```python
from build123d import *

# Parameters (mm, degrees)
SKETCH1_R           = 150
BOSS_EXTRUDE1_DEPTH = 9.52
SKETCH2_R           = 15.5
CUT_EXTRUDE1_DEPTH  = 213.345544808
SKETCH3_R           = 17.505
CUT_EXTRUDE2_DEPTH  = 8
SKETCH4_R           = 2.5
SKETCH4_R_2         = 1.65
CUT_EXTRUDE3_DEPTH  = 213.345544808
SKETCH6_R           = 1.65
CUT_EXTRUDE5_DEPTH  = 213.345544808
SKETCH7_R           = 4.5
CUT_EXTRUDE6_DEPTH  = 213.345544808


with BuildPart() as part:
    # Sketch1 → Boss-Extrude1 (new body)
    with BuildSketch(Plane(origin=(0, 0, 0), x_dir=(1, 0, 0), z_dir=(0, 1, 0))):
        with Locations(Location((0, 0, 0), (0, 0, 270))):
            Circle(SKETCH1_R)
    extrude(amount=BOSS_EXTRUDE1_DEPTH)

    # Sketch2 → Cut-Extrude1 (cut, through all)
    with BuildSketch(Plane(origin=(0, 9.52, 0), x_dir=(1, 0, 0), z_dir=(0, 1, 0))):
        with Locations(Location((0, 0, 0), (0, 0, 270))):
            Circle(SKETCH2_R)
    extrude(amount=-CUT_EXTRUDE1_DEPTH, mode=Mode.SUBTRACT)

    # Sketch3 → Cut-Extrude2 (cut)
    with BuildSketch(Plane(origin=(0, 9.52, 0), x_dir=(1, 0, 0), z_dir=(0, 1, 0))):
        with Locations(Location((0, 0, 0), (0, 0, 270))):
            Circle(SKETCH3_R)
    extrude(amount=-CUT_EXTRUDE2_DEPTH, mode=Mode.SUBTRACT)

    # Sketch4 → Cut-Extrude3 (cut, through all)
    with BuildSketch(Plane(origin=(0, 9.52, 0), x_dir=(1, 0, 0), z_dir=(0, 1, 0))):
        with Locations(Location((10.725147849, -21.193217308, 0), (0, 0, 270))):
            Circle(SKETCH4_R)
        with Locations(Location((-23.716438501, 1.308358157, 0), (0, 0, 270))):
            Circle(SKETCH4_R)
        with Locations(Location((12.991290652, 19.884859151, 0), (0, 0, 270))):
            Circle(SKETCH4_R)
        with Locations(Location((67.75, -117.346442213, 0), (0, 0, 270))):
            Circle(SKETCH4_R_2)
        with Locations(Location((0, -135.5, 0), (0, 0, 270))):
            Circle(SKETCH4_R_2)
        with Locations(Location((-67.75, -117.346442213, 0), (0, 0, 270))):
            Circle(SKETCH4_R_2)
        with Locations(Location((-117.346442213, -67.75, 0), (0, 0, 270))):
            Circle(SKETCH4_R_2)
        with Locations(Location((-135.5, 0, 0), (0, 0, 270))):
            Circle(SKETCH4_R_2)
        with Locations(Location((-117.346442213, 67.75, 0), (0, 0, 270))):
            Circle(SKETCH4_R_2)
        with Locations(Location((-67.75, 117.346442213, 0), (0, 0, 270))):
            Circle(SKETCH4_R_2)
        with Locations(Location((0, 135.5, 0), (0, 0, 270))):
            Circle(SKETCH4_R_2)
        with Locations(Location((67.75, 117.346442213, 0), (0, 0, 270))):
            Circle(SKETCH4_R_2)
        with Locations(Location((117.346442213, 67.75, 0), (0, 0, 270))):
            Circle(SKETCH4_R_2)
        with Locations(Location((135.5, 0, 0), (0, 0, 270))):
            Circle(SKETCH4_R_2)
        with Locations(Location((117.346442213, -67.75, 0), (0, 0, 270))):
            Circle(SKETCH4_R_2)
    extrude(amount=-CUT_EXTRUDE3_DEPTH, mode=Mode.SUBTRACT)

    # Sketch6 → Cut-Extrude5 (cut, through all)
    with BuildSketch(Plane(origin=(0, 0, 0), x_dir=(-1, 0, 0), z_dir=(0, -1, 0))):
        with Locations(Location((-63.964762127, 126.790217897, 0), (0, 0, 90))):
            Circle(SKETCH6_R)
        with Locations(Location((-77.821168587, 118.790217897, 0), (0, 0, 90))):
            Circle(SKETCH6_R)
        with Locations(Location((-64.892965357, 112.397913052, 0), (0, 0, 90))):
            Circle(SKETCH6_R)
        with Locations(Location((-9.698914748, 129.423022928, 0), (0, 0, 90))):
            Circle(SKETCH6_R)
        with Locations(Location((-2.618045494, 141.987309243, 0), (0, 0, 90))):
            Circle(SKETCH6_R)
        with Locations(Location((-18.573306249, 140.791627746, 0), (0, 0, 90))):
            Circle(SKETCH6_R)
        with Locations(Location((59.247207157, 129.062072633, 0), (0, 0, 90))):
            Circle(SKETCH6_R)
        with Locations(Location((44.353227178, 134.907529023, 0), (0, 0, 90))):
            Circle(SKETCH6_R)
        with Locations(Location((47.416124875, 120.814315845, 0), (0, 0, 90))):
            Circle(SKETCH6_R)
        with Locations(Location((109.377823811, 90.574509696, 0), (0, 0, 90))):
            Circle(SKETCH6_R)
        with Locations(Location((98.495060007, 102.303339645, 0), (0, 0, 90))):
            Circle(SKETCH6_R)
        with Locations(Location((95.139819447, 88.276851818, 0), (0, 0, 90))):
            Circle(SKETCH6_R)
        with Locations(Location((133.128738238, 49.436719183, 0), (0, 0, 90))):
            Circle(SKETCH6_R)
        with Locations(Location((124.019905964, 38.255074644, 0), (0, 0, 90))):
            Circle(SKETCH6_R)
        with Locations(Location((137.844821028, 34.14755429, 0), (0, 0, 90))):
            Circle(SKETCH6_R)
        with Locations(Location((141.394637144, -13.221449816, 0), (0, 0, 90))):
            Circle(SKETCH6_R)
        with Locations(Location((128.3363291, -19.343589231, 0), (0, 0, 90))):
            Circle(SKETCH6_R)
        with Locations(Location((139.009960885, -29.042743035, 0), (0, 0, 90))):
            Circle(SKETCH6_R)
        with Locations(Location((121.655594073, -73.260948528, 0), (0, 0, 90))):
            Circle(SKETCH6_R)
        with Locations(Location((112.642473144, -86.480768917, 0), (0, 0, 90))):
            Circle(SKETCH6_R)
        with Locations(Location((107.234168316, -73.111018025, 0), (0, 0, 90))):
            Circle(SKETCH6_R)
        with Locations(Location((64.892965357, -112.397913052, 0), (0, 0, 90))):
            Circle(SKETCH6_R)
        with Locations(Location((63.964762127, -126.790217897, 0), (0, 0, 90))):
            Circle(SKETCH6_R)
        with Locations(Location((77.821168587, -118.790217897, 0), (0, 0, 90))):
            Circle(SKETCH6_R)
        with Locations(Location((9.698914748, -129.423022928, 0), (0, 0, 90))):
            Circle(SKETCH6_R)
        with Locations(Location((2.618045494, -141.987309243, 0), (0, 0, 90))):
            Circle(SKETCH6_R)
        with Locations(Location((18.573306249, -140.791627746, 0), (0, 0, 90))):
            Circle(SKETCH6_R)
        with Locations(Location((-44.353227178, -134.907529023, 0), (0, 0, 90))):
            Circle(SKETCH6_R)
        with Locations(Location((-59.247207157, -129.062072633, 0), (0, 0, 90))):
            Circle(SKETCH6_R)
        with Locations(Location((-47.416124875, -120.814315845, 0), (0, 0, 90))):
            Circle(SKETCH6_R)
        with Locations(Location((-98.495060007, -102.303339645, 0), (0, 0, 90))):
            Circle(SKETCH6_R)
        with Locations(Location((-109.377823811, -90.574509696, 0), (0, 0, 90))):
            Circle(SKETCH6_R)
        with Locations(Location((-95.139819447, -88.276851818, 0), (0, 0, 90))):
            Circle(SKETCH6_R)
        with Locations(Location((-124.019905964, -38.255074644, 0), (0, 0, 90))):
            Circle(SKETCH6_R)
        with Locations(Location((-137.844821028, -34.14755429, 0), (0, 0, 90))):
            Circle(SKETCH6_R)
        with Locations(Location((-133.128738238, -49.436719183, 0), (0, 0, 90))):
            Circle(SKETCH6_R)
        with Locations(Location((-128.3363291, 19.343589231, 0), (0, 0, 90))):
            Circle(SKETCH6_R)
        with Locations(Location((-141.394637144, 13.221449816, 0), (0, 0, 90))):
            Circle(SKETCH6_R)
        with Locations(Location((-139.009960885, 29.042743035, 0), (0, 0, 90))):
            Circle(SKETCH6_R)
        with Locations(Location((-107.234168316, 73.111018025, 0), (0, 0, 90))):
            Circle(SKETCH6_R)
        with Locations(Location((-121.655594073, 73.260948528, 0), (0, 0, 90))):
            Circle(SKETCH6_R)
        with Locations(Location((-112.642473144, 86.480768917, 0), (0, 0, 90))):
            Circle(SKETCH6_R)
    extrude(amount=-CUT_EXTRUDE5_DEPTH, mode=Mode.SUBTRACT)

    # Sketch7 → Cut-Extrude6 (cut, through all)
    with BuildSketch(Plane(origin=(0, 9.52, 0), x_dir=(1, 0, 0), z_dir=(0, 1, 0))):
        with Locations(Location((-60, -60, 0), (0, 0, 270))):
            Circle(SKETCH7_R)
        with Locations(Location((60, -60, 0), (0, 0, 270))):
            Circle(SKETCH7_R)
        with Locations(Location((60, 60, 0), (0, 0, 270))):
            Circle(SKETCH7_R)
        with Locations(Location((-60, 60, 0), (0, 0, 270))):
            Circle(SKETCH7_R)
    extrude(amount=-CUT_EXTRUDE6_DEPTH, mode=Mode.SUBTRACT)


solid = part.part
```
The model under review builds one solid part; all positions refer to its coordinate system, in mm. A direction names the side the tool comes from. Give positions to 0.01 mm unless a question says otherwise; leave off trailing zeros. Order: outer loops, then holes, each group sorted by start corner. A loop starts at its lowest first (then second) coordinate and runs counter-clockwise, first axis right, second up. Notation, with made-up numbers: (-4, 14.25) - (50, 14.25) arc R22 ccw to (50, 32.25) - close; hole circle Ø9 at (74.25, -34.75). An arc over 180 degrees is marked (long way). Use CSV: the item, a comma, the result in double quotes. Start each with the question number.
Q1. We need section A-A, the plane z = 60. Write out the cut boundary in (x, y).
Q2. Tool access review of faces 1 (the cylindrical face through (17.356, 5.576, -2.279)), 2 (the cylindrical face through (61.352, 4.827, -55.708)): name each direction out of +Z, -Z, +X, -X, +Y, -Y from which nothing blocks a thin tool from reaching the whole face with its end or side.
Q3. We need section B-B, the plane y = 4.5. State how many separate pieces and enclosed holes the cut face has, and give its area (3 significant figures).
Q4. To check wall thickness, follow line 1 along X through (y, z) = (5.5, 86.5); line 2 along X through (y, z) = (4.5, 135.5); line 3 along X through (y, z) = (3.25, -135.5). State the ranges of each line that lie inside material, in increasing order. Write a range as [from, to].
Q5. Clearance check with flat-ended pins moving along their axes: pin 1 Ø5 at (x, y) = (-27, 1.5) entering from +Z; pin 2 Ø1.5 at (x, y) = (15.5, 2) entering from -Z; pin 3 Ø1 at (y, z) = (3.5, -17) entering from +X; pin 4 Ø2 at (x, z) = (-64.89, 112.4) entering from -Y. State where each tip first meets the part, or that it passes through.
Q6. We need section C-C, the plane x = -84.5. Write out the cut boundary in (y, z), and give its area (3 significant figures).
Q7. The part is to be moulded in two halves that separate along Z. For faces 3 (the cylindrical face through (-61.72, 4.83, -55.84)), 4 (the flat face through (2, 9.52, 31)), 5 (the cylindrical face through (-91.273, 4.693, -119.035)), 6 (the cylindrical face through (15.368, 0.771, -2.018)), say which applies: +Z half, -Z half, draft (parallel to the pull), parting line (faces both ways), or undercut.
Outcome:
1,outline,"(-137.48, 0) - (-64.5, 0) - (-64.5, 9.52) - (-137.48, 9.52) - close; (-55.5, 0) - (55.5, 0) - (55.5, 9.52) - (-55.5, 9.52) - close; (64.5, 0) - (137.48, 0) - (137.48, 9.52) - (64.5, 9.52) - close"
2,face 1,"+Y"
2,face 2,"+Y, -Y"
3,separate pieces,"1"
3,enclosed holes,"62"
3,area,"68,900 mm^2"
4,line 1,"x = [-122.55, -114.29], [-110.99, 122.55]"
4,line 2,"x = [-64.34, -1.65], [1.65, 42.81], [45.89, 64.34]"
4,line 3,"x = [-64.34, -45.89], [-42.81, -1.65], [1.65, 64.34]"
5,pin 1,"stops at z = 147.99"
5,pin 2,"stops at z = -149.27"
5,pin 3,"stops at x = 149.09"
5,pin 4,"passes through"
6,outline,"(0, -123.93) - (9.52, -123.93) - (9.52, 123.93) - (0, 123.93) - close"
6,area,"2,360 mm^2"
7,face 3,"undercut"
7,face 4,"draft"
7,face 5,"parting line"
7,face 6,"undercut"
